```python
from build123d import *

# Parameters (mm, degrees)
SKETCH_W     = 50
SKETCH_H     = 100
PAD_DEPTH    = 3
SKETCH001_R  = 1.6
POCKET_DEPTH = 3
FILLET_R     = 1


with BuildPart() as part:
    # Sketch → Pad (new body)
    with BuildSketch(Plane.XY):
        Rectangle(SKETCH_W, SKETCH_H)
    extrude(amount=PAD_DEPTH)

    # Sketch001 (on Face6 of Pad) → Pocket (cut)
    with BuildSketch(Plane.XY.offset(3)):
        with Locations((-21, 46)):
            Circle(SKETCH001_R)
        with Locations((21, 46)):
            Circle(SKETCH001_R)
        with Locations((-21, -46)):
            Circle(SKETCH001_R)
        with Locations((21, -46)):
            Circle(SKETCH001_R)
    extrude(amount=-POCKET_DEPTH, mode=Mode.SUBTRACT)

    # Fillet
    fillet_edges = [part.edges().sort_by_distance(p)[0] for p in [
        (-25, 50, 1.5),
        (25, 50, 1.5),
        (25, -50, 1.5),
        (-25, -50, 1.5),
    ]]
    fillet(fillet_edges, radius=FILLET_R)


solid = part.part
```
Geometry: final body of the model. Coordinates: model frame, mm. Coordinates: 2 decimals unless noted, no trailing zeros. Loops run counter-clockwise (first coordinate to the right, second up) from the corner with the lowest first, then second, coordinate; pieces in that order, holes last. Notation, with made-up numbers: M 2,13.5 L 51,13.5 A18 cw 51,35.5 Z; hole C 29.5,-35.75 d1. An arc over 180 degrees is marked long. Put each result on its own line as item: value.
(1) Cut plane A-A on x = 21. Return the cut outline in (y, z), then the cut area to 3 significant figures.
Answer sheet:
outline: M -50,0 L -47.6,0 L -47.6,3 L -50,3 Z; M -44.4,0 L 44.4,0 L 44.4,3 L -44.4,3 Z; M 47.6,0 L 50,0 L 50,3 L 47.6,3 Z
area: 281 mm^2
(2) Draft query along X for faces 1 (the face through (21.74, -47.42, 1.52)), 2 (the face through (-25, -1, 1)), 3 (the face through (25, -1, 1)). Return one class per face: pulls with the +X half, pulls with the -X half, needs draft (parallel to the pull), parting line crosses it, or undercut.
Answer sheet:
face 1: undercut
face 2: pulls with the -X half
face 3: pulls with the +X half
(3) First-contact query: pin 1 (3 mm diameter, centred on x = -6, y = 14, fed in from -Z). Flat tip, straight axial feed; report the tip coordinate or a pass-through.
Answer sheet:
pin 1: stops at z = 0
(4) Cut plane B-B on y = 46. Return the cut outline in (x, z), then the cut area to 3 significant figures.
Answer sheet:
outline: M -25,0 L -22.6,0 L -22.6,3 L -25,3 Z; M -19.4,0 L 19.4,0 L 19.4,3 L -19.4,3 Z; M 22.6,0 L 25,0 L 25,3 L 22.6,3 Z
area: 131 mm^2
(5) Material intervals for probe 1 along Y at (x, z) = (21, 1.6); probe 2 along Y at (x, z) = (20, 0.55), sorted ascending.
Answer sheet:
probe 1: y = -50 to -47.6, -44.4 to 44.4, 47.6 to 50
probe 2: y = -50 to -47.25, -44.75 to 44.75, 47.25 to 50
